Design review of the part built by this model. Coordinates are the model's own, in mm. A direction names the side the tool comes from. Round coordinates to 2 decimals unless told otherwise and drop trailing zeros. Write each loop counter-clockwise with the first axis right and the second up, starting at its lowest first coordinate (ties: lowest second). Pieces come first, ordered by that corner, then holes. Notation, with made-up numbers: (-4.75, -4.75) -> (14.25, -4.75) arc R13 cw to (14.25, 7.25) -> close; hole circle Ø1 at (76, -38). An arc over 180 degrees is marked (long way). Write item = value, one per line. Start each with the question number.
Item 1: Add section A-A, the plane z = 35.5. State the section outline as (x, y) points.
Item 2: For pin 1 Ø3 at (x, z) = (-119.5, 58) entering from +Y; pin 2 Ø3 at (x, z) = (-54, 51.5) entering from +Y; pin 3 Ø2 at (x, z) = (-119.5, 59) entering from -Y, all flat-tipped, find the tip position at first contact; note any pin that passes through.
Item 3: Add section B-B, the plane y = 1271.5. State the section outline as (x, z) points, then the cut area to 3 significant figures.
Item 4: Mouldability with a two-part tool opening along Z and no side actions: class faces 1 (the flat face through (-118.181, 943, 49)), 2 (the flat face through (-122.181, 945, 49)), 3 (the flat face through (-88, 956, 13.326)), 4 (the flat face through (-87, 984, 79.326)) as released by +Z, released by -Z, zero draft, split by the parting line, or undercut.
Item 5: To check wall thickness, follow L1, parallel to Z at x = -71, y = 609.5; L2, parallel to X at y = 707, z = 40; L3, parallel to X at y = 1890, z = 81.65. State the ranges of each line that lie inside material, in increasing order.
Item 6: Machinability: for faces 5 (the flat face through (-52.181, 956, 48)), 6 (the flat face through (-56.181, 952, 48)), which of the approach directions +Z, -Z, +X, -X, +Y, -Y give a long, thin tool a straight path to every point of the face, cutting with its end or side? Answer none if there is none.
Solid Edge part; units mm, degrees
sketch "Sketch1" plane through (0, 0, 0) normal (0, -1, 0) x (1, 0, 0)
  line L0 (-122.1808, 13.3262) -> (-52.1808, 13.3262)
  line L1 (-52.1808, 13.3262) -> (-52.1808, 83.3262)
  line L2 (-52.1808, 83.3262) -> (-122.1808, 83.3262)
  line L3 (-122.1808, 83.3262) -> (-122.1808, 13.3262)
  line L4 (-118.1808, 17.3262) -> (-56.1808, 17.3262)
  line L5 (-56.1808, 17.3262) -> (-56.1808, 79.3262)
  line L6 (-56.1808, 79.3262) -> (-118.1808, 79.3262)
  line L7 (-118.1808, 79.3262) -> (-118.1808, 17.3262)
  dimension "D1" = 122.1808
  dimension "D2" = 52.1808
  dimension "D3" = 122.1808
extrude "Protrusion1" add sketch "Sketch1" against normal blind 1940
sketch "Sketch2" plane through (-87.1808, 1079, 13.3262) normal (0, 0, -1) x (0, -1, 0)
  circle A0 centre (-811, 0) radius 6.1
  circle A1 centre (-841, 0) radius 6.1
  circle A2 centre (1059, 0) radius 6.1
  dimension "D1" = 1059
  dimension "D2" = 841
extrude "Cutout1" cut sketch "Sketch2" against normal through all
sketch "Sketch3" plane through (-52.1808, 1079, 63.3262) normal (1, 0, 0) x (0, -1, 0)
  line L0 (1034, -16) -> (1079, -16)
  line L1 (1079, -16) -> (1079, 46)
  line L2 (1079, 46) -> (1034, 46)
  line L3 (1034, 46) -> (1034, -16)
  line L4 (-861, -16) -> (-806, -16)
  line L5 (-806, -16) -> (-806, 46)
  line L6 (-806, 46) -> (-861, 46)
  line L7 (-861, 46) -> (-861, -16)
  dimension "D1" = 806
  dimension "D2" = 806
  dimension "D3" = 1034
  dimension "D4" = 1034
extrude "Cutout2" cut sketch "Sketch3" against normal up to next
sketch "Sketch4" plane through (-92.1808, 1005.1, 13.3262) normal (0, 0, -1) x (0, -1, 0)
  line L0 (-934.9, 30) -> (-909.9, 30)
  line L1 (-909.9, 30) -> (-934.9, 0.2062)
  line L2 (-934.9, 0.2062) -> (-934.9, 30)
  dimension "D1" = 934.9
extrude "Cutout3" cut sketch "Sketch4" against normal through all
sketch "Sketch5" plane through (-92.1808, 1005.1, 13.3262) normal (0, 0, -1) x (0, 1, 0)
  line L0 (-1005.1, -29) -> (-1004.2609, -30)
  line L1 (-1004.2609, -30) -> (-1005.1, -30)
  line L2 (-1005.1, -30) -> (-1005.1, -29)
  dimension "D1" = 1005.1
extrude "Cutout4" cut sketch "Sketch5" against normal through all
sketch "Sketch6" plane through (-122.1808, 957.9195, 48.3262) normal (-1, 0, 0) x (0, -1, 0)
  line L0 (-982.0805, -31) -> (-882.0805, -31)
  line L1 (-882.0805, -31) -> (-882.0805, 31)
  line L2 (-882.0805, 31) -> (-982.0805, 31)
  line L3 (-982.0805, 31) -> (-982.0805, -31)
  dimension "D1" = 982.0805
  dimension "D2" = 882.0805
extrude "Cutout5" cut sketch "Sketch6" against normal up to next
sketch "Sketch7" plane through (-122.1808, 957.9195, 48.3262) normal (-1, 0, 0) x (0, 1, 0)
  line L0 (-957.9195, -31) -> (-887.9195, -31)
  line L1 (-887.9195, -31) -> (-887.9195, 31)
  line L2 (-887.9195, 31) -> (-957.9195, 31)
  line L3 (-957.9195, 31) -> (-957.9195, -31)
  dimension "D1" = 957.9195
  dimension "D2" = 887.9195
extrude "Cutout6" cut sketch "Sketch7" against normal up to next
fillet "Round1" radius 5 4 edges at (-54.1808, 45, 79.3262) (-54.1808, 45, 17.3262) (-54.1808, 1885, 79.3262) (-54.1808, 1885, 17.3262)
properties material "Aluminum, 6061-T6"
Result set:
q1.outline = (-122.18, 70) -> (-118.18, 70) -> (-118.18, 1840) -> (-122.18, 1840) -> close; (-56.18, 45) -> (-52.18, 45) -> (-52.18, 1885) -> (-56.18, 1885) -> close
q2.pin_1 = 1840
q2.pin_2 = 1885
q2.pin_3 = 70
q3.outline = (-122.18, 13.33) -> (-52.18, 13.33) -> (-52.18, 83.33) -> (-122.18, 83.33) -> close; hole (-118.18, 17.33) -> (-56.18, 17.33) -> (-56.18, 79.33) -> (-118.18, 79.33) -> close
q3.area = 1,060 mm²
q4.face_1 = undercut
q4.face_2 = zero draft
q4.face_3 = released by -Z
q4.face_4 = undercut
q5.L1 = 13.33 to 17.33, 79.33 to 83.33
q5.L2 = -122.18 to -118.18, -56.18 to -52.18
q5.L3 = -122.18 to -93.28, -81.08 to -52.18
q6.face_5 = +Z, -Z, +X, +Y, -Y
q6.face_6 = +Y, -Y
